from build123d import *

# Parameters (mm, degrees)
F0_W      = 50.8
F0_H      = 31.75
F1_DEPTH  = 31.75
F3_DEPTH  = 12.7
F4_DEPTH  = 19.05
F6_DEPTH  = 19.05
F8_DEPTH  = 31.75
F10_DEPTH = 19.05


with BuildPart() as f1:
    # F0 (on Front) → F1 (new body)
    with BuildSketch(Plane.XZ):
        with Locations((25.4, 15.875)):
            Rectangle(F0_W, F0_H)
    extrude(amount=F1_DEPTH)

    # F2 (on face) → F3 (cut)
    with BuildSketch(Plane.XZ.offset(31.75)):
        Polygon((50.8, 31.75), (38.1, 31.75), (50.8, 15.875), align=None)
    extrude(amount=-F3_DEPTH, mode=Mode.SUBTRACT)

    # F4 (cut): a face of the model
    f4_faces = [f1.faces().sort_by_distance(p)[0] for p in [
        (46.5666666667, -19.05, 26.4583333333),
    ]]
    extrude(f4_faces, amount=-F4_DEPTH, mode=Mode.SUBTRACT)

    # F5 (on face) → F6 (cut)
    with BuildSketch(Plane.XZ.offset(31.75)):
        Polygon((38.1, 31.75), (31.75, 31.75), (31.75, 15.875), (50.8, 15.875), align=None)
    extrude(amount=-F6_DEPTH, mode=Mode.SUBTRACT)

    # F7 (on face) → F8 (cut)
    with BuildSketch(Plane.YZ.offset(31.75)):
        Polygon((-31.75, 15.875), (-12.7, 31.75), (-31.75, 31.75), align=None)
    extrude(amount=-F8_DEPTH, mode=Mode.SUBTRACT)

    # F9 (on face) → F10 (cut)
    with BuildSketch(Plane(origin=(0, 0, 0), x_dir=(0, -1, 0), z_dir=(-1, 0, 0))):
        Polygon((31.75, 15.875), (12.7, 31.75), (12.7, 15.875), align=None)
    extrude(amount=-F10_DEPTH, mode=Mode.SUBTRACT)


solid = f1.part
Here's how the part is built. I have some questions about the finished solid (model axes, mm). A direction names the side the tool comes from. Coordinates: 2 decimals unless noted, no trailing zeros. Loops run counter-clockwise (first coordinate to the right, second up) from the corner with the lowest first, then second, coordinate; pieces in that order, holes last.
1. Imagine slicing it at A-A, the plane z = 30.5. Please give me the cut outline in (x, y), and give its area (3 significant figures).
2. Imagine slicing it at D-D, the plane y = -4. Please give me the cut outline in (x, z) (3 decimals), and give its area (3 significant figures).
3. I need wall thicknesses on L1, parallel to Z at x = 3.5, y = -18 (3 decimals); L2, parallel to Y at x = 42.5, z = 17; L3, parallel to X at y = -23, z = 20.5. Which ranges of each line are inside material? Lowest first, please.
4. For P1, Ø2, axis at x = 34.5, z = 16, coming from the +Y side; P2, Ø8, axis at x = 5, z = 22, coming from the -Y side; P3, Ø3, axis at x = 13, y = -18, coming from the +Z side (3 decimals); P4, Ø8, axis at y = -25, z = 23, coming from the +X side, each with a flat end and sliding along its axis, tell me the tip position at first contact or that it passes through.
5. Imagine slicing it at C-C, the plane y = -17.5. Please give me the cut outline in (x, z) (3 decimals), and give its area (3 significant figures).
6. Imagine slicing it at B-B, the plane x = 30. Please give me the cut outline in (y, z) (3 decimals).
7. For faces 1 (the flat face through (9, -12.7, 24)), 2 (the flat face through (39, -12.7, 22)), 3 (the flat face through (25, -22, 24)), which set-ups out of +Z, -Z, +X, -X, +Y, -Y let a thin tool reach every point of the face, with its end or its side?
Taken from the geometry:
1. outline: (0, -12.7) - (19.05, -12.7) - (19.05, -14.2) - (31.75, -14.2) - (31.75, -12.7) - (39.1, -12.7) - (39.1, 0) - (0, 0) - close
1. area: 516 mm2
2. outline: (0, 0) - (50.8, 0) - (50.8, 15.875) - (38.1, 31.75) - (0, 31.75) - close
2. area: 1,510 mm2
3. L1: z = 0 to 15.875
3. L2: y = -12.7 to 0
3. L3: x = 19.05 to 31.75
4. P1: stops at y = 0
4. P2: stops at y = -12.7
4. P3: stops at z = 15.875
4. P4: stops at x = 31.75
5. outline: (0, 0) - (50.8, 0) - (50.8, 15.875) - (31.75, 15.875) - (31.75, 27.75) - (19.05, 27.75) - (19.05, 15.875) - (0, 15.875) - close
5. area: 957 mm2
6. outline: (-31.75, 0) - (0, 0) - (0, 31.75) - (-12.7, 31.75) - (-31.75, 15.875) - close
7. face 1: +Z, -X, -Y
7. face 2: +Z, +X, -Y
7. face 3: +Z, +X, -X, -Y
